```python
from build123d import *

# Parameters (mm, degrees)
SKETCH_1_R      = 20
SKETCH_1_R_2    = 14
EXTRUDE_1_DEPTH = 100
SKETCH_2_W      = 1.7
SKETCH_2_H      = 30


with BuildPart() as part:
    # Эскиз1 → Вытянуть-Тонкостенный1 (new body)
    with BuildSketch(Plane(origin=(0, 0, 0), x_dir=(1, 0, 0), z_dir=(0, 1, 0))):
        Circle(SKETCH_1_R)
        Circle(SKETCH_1_R_2, mode=Mode.SUBTRACT)
    extrude(amount=EXTRUDE_1_DEPTH)

    # Эскиз2 → Вырез-Повернуть1 (revolve, cut)
    with BuildSketch(Plane(origin=(0, 0, 0), x_dir=(0, 0, -1), z_dir=(1, 0, 0))):
        with Locations((19.15, 15)):
            Rectangle(SKETCH_2_W, SKETCH_2_H)
        Polygon((17, 100), (17.749980471, 40.001562317), (20, 40.001562317), (20, 100), align=None)
    revolve(axis=Axis((0, -5.85508708, 0), (0, 1, 0)), mode=Mode.SUBTRACT)


solid = part.part
```
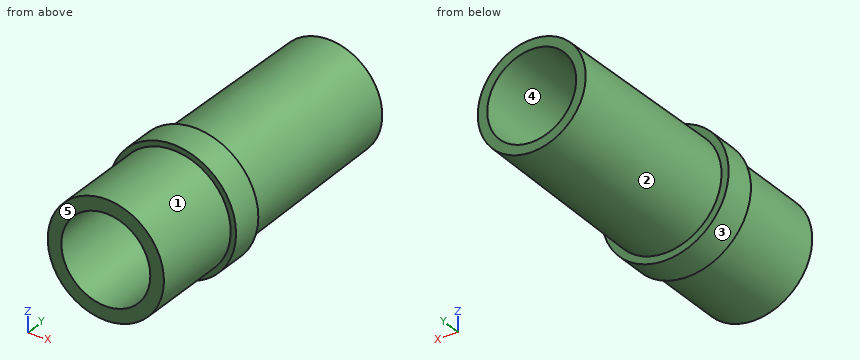
Can you work these out from the model? Positions are in its coordinate system, mm. Face numbers are marked on the shaded views. A direction names the side the tool comes from. Coordinates: 2 decimals unless noted, no trailing zeros. Order: outer loops, then holes, each group sorted by start corner. A loop starts at its lowest first (then second) coordinate and runs counter-clockwise, first axis right, second up.
1. I need wall thicknesses on line 1 (X direction, y = 29.5, z = 0); line 2 (Z direction, x = 0, y = 36.5); line 3 (Y direction, x = 16, z = -10.5). Which ranges of each line are inside material? Lowest first, please.
2. If we section it at B-B (y = 84.5): Please give me the cut outline in (x, z), then the cut area to 3 significant figures.
3. If we section it at A-A (y = 6): Please give me the cut outline in (x, z).
4. Thinking about a two-plate mould opening in Z: for the marked faces 3, 4 and 5, which applies, +Z half, -Z half, draft (parallel to the pull), parting line (faces both ways), or undercut?
5. I'm going to push flat-ended pins straight in: pin 1 (2 mm diameter, centred on y = 32.5, z = -16, fed in from -X); pin 2 (6 mm diameter, centred on y = 49.5, z = -8.5, fed in from +X); pin 3 (12 mm diameter, centred on x = 4, y = 62.5, fed in from -Z); pin 4 (20 mm diameter, centred on x = 6.5, z = -0.5, fed in from +Y). Where does each tip first touch, or does it pass through?
6. For the marked faces 1 and 2, which set-ups out of +Z, -Z, +X, -X, +Y, -Y let a thin tool reach every point of the face, with its end or its side?
Entries:
1. line 1: x = -18.3 to -14, 14 to 18.3
1. line 2: z = -20 to -14, 14 to 20
1. line 3: y = 30 to 40
2. outline: circle Ø34.39 at (0, 0); hole circle Ø28 at (0, 0)
2. area: 313 mm2
3. outline: circle Ø36.6 at (0, 0); hole circle Ø28 at (0, 0)
4. face 3: parting line
4. face 4: undercut
4. face 5: draft
5. pin 1: stops at x = -13.23
5. pin 2: stops at x = 16.75
5. pin 3: stops at z = -17.53
5. pin 4: stops at y = 100
6. face 1: -Y
6. face 2: +Y
